The listing builds one solid part. Answer for the finished solid, in the listing's coordinates (mm). A direction names the side the tool comes from. Coordinates: 2 decimals unless noted, no trailing zeros. Loops run counter-clockwise (first coordinate to the right, second up) from the corner with the lowest first, then second, coordinate; pieces in that order, holes last. Notation, with made-up numbers: M 78,53.5 L 96,53.5 A13 cw 96,62.5 Z; hole C 16.5,-15.5 d1. An arc over 180 degrees is marked long. Return JSON: item names as keys, results as strings. Group by question number.
1. Which of the six approach directions +Z, -Z, +X, -X, +Y, -Y give full straight-line access (tool end or side, diameter ignored) to faces 4 (the face through (-0.785, -3.199, -5.424)), 5 (the face through (-0.785, 3.199, -5.407)), 6 (the face through (0.5, 0, -5.5))?
2. Section B-B (x = 4.5) is taken. Write down the section's boundary in (y, z), then the cut area to 3 significant figures.
3. Section A-A (z = 0) is taken. Write down the section's boundary in (x, y).
4. Section D-D (y = -0.5) is taken. Write down the section's boundary in (x, z), then the cut area to 3 significant figures.
5. Straight lines are drawn through the part: L1, parallel to X at y = 0.5, z = 0; L2, parallel to X at y = 2, z = 4.5; L3, parallel to Z at x = -2.5, y = 1.5. For each, find the intervals that lie inside material, in ascending order. Write a range as from..to.
6. Section C-C (x = 0) is taken. Write down the section's boundary in (y, z), then the cut area to 3 significant figures.
7. Given P1, Ø1, axis at y = -2.5, z = -4, coming from the -X side; P2, Ø0.8, axis at y = 1, z = -5.5, coming from the -X side; P3, Ø0.5, axis at y = -0.5, z = -5.5, coming from the +X side; P4, Ø1.5, axis at x = 3.5, z = -1, coming from the +Y side, each flat-ended and moving along its own axis, determine where each tip first touches the part or whether it passes through.
8. The mould has two halves that part along Z. Classify faces 1 (the face through (-0.259, 0.049, 6.034)), 2 (the face through (-0.215, -0.049, 5.035)), 3 (the face through (-0.5, 0, -5.5)): pulls with the +Z half, pulls with the -Z half, needs draft (parallel to the pull), parting line crosses it, or undercut.
```python
from build123d import *

# Parameters (mm, degrees)
SKETCH3_R               = 6.04
SKETCH3_R_2             = 5.04
EXTRUDE_THIN1_DEPTH     = 3.5
SKETCH4_W               = 1
SKETCH4_H               = 1000
CUT_EXTRUDE1_DEPTH      = 4.5
CUT_EXTRUDE1_DEPTH_BACK = 4.5
FILLET1_R               = 1


with BuildPart() as part:
    # Sketch3 → Extrude-Thin1 (new body, symmetric)
    with BuildSketch(Plane(origin=(0, 0, 0), x_dir=(1, 0, 0), z_dir=(0, 1, 0))):
        Circle(SKETCH3_R)
        Circle(SKETCH3_R_2, mode=Mode.SUBTRACT)
    extrude(amount=EXTRUDE_THIN1_DEPTH, both=True)

    # Sketch4 → Cut-Extrude1 (cut, two sides)
    with BuildSketch(Plane(origin=(0, 0, 0), x_dir=(1, 0, 0), z_dir=(0, 1, 0))) as cut_extrude1_sk:
        with Locations((0, 500)):
            Rectangle(SKETCH4_W, SKETCH4_H)
    extrude(amount=CUT_EXTRUDE1_DEPTH, mode=Mode.SUBTRACT)
    extrude(cut_extrude1_sk.sketch, amount=-CUT_EXTRUDE1_DEPTH_BACK, mode=Mode.SUBTRACT)

    # Fillet1
    fillet1_edges = [part.edges().sort_by_distance(p)[0] for p in [
        (0.5, -3.5, -5.517203073),
        (-0.5, -3.5, -5.517203073),
        (0.5, 3.5, -5.517203073),
        (-0.5, 3.5, -5.517203073),
    ]]
    fillet(fillet1_edges, radius=FILLET1_R)


solid = part.part
```
Worked out:
{
 "1": {"face 4": "-Z, -Y", "face 5": "-Z, +Y", "face 6": "-Z, +Y, -Y"},
 "2": {"outline": "M -3.5,-4.03 L 3.5,-4.03 L 3.5,-2.27 L -3.5,-2.27 Z; M -3.5,2.27 L 3.5,2.27 L 3.5,4.03 L -3.5,4.03 Z", "area": "24.6 mm^2"},
 "3": {"outline": "M -6.04,-3.5 L -5.04,-3.5 L -5.04,3.5 L -6.04,3.5 Z; M 5.04,-3.5 L 6.04,-3.5 L 6.04,3.5 L 5.04,3.5 Z"},
 "4": {"outline": "M -0.5,-6.02 L -0.5,-5.02 A5.04 cw long 0.5,-5.02 L 0.5,-6.02 A6.04 ccw long Z", "area": "33.8 mm^2"},
 "5": {"L1": "-6.04..-5.04, 5.04..6.04", "L2": "-4.03..-2.27, 2.27..4.03", "L3": "-5.5..-4.38, 4.38..5.5"},
 "6": {"outline": "M -3.5,5.04 L 3.5,5.04 L 3.5,6.04 L -3.5,6.04 Z", "area": "7.00 mm^2"},
 "7": {"P1": "x = -4.92", "P2": "x = -3.24", "P3": "x = 2.99", "P4": "through"},
 "8": {"face 1": "parting line crosses it", "face 2": "undercut", "face 3": "needs draft"}
}
